CAD build for the part. Positions are in the model's coordinates, mm. A direction names the side the tool comes from. Coordinates: 2 decimals unless noted, no trailing zeros. Order: outer loops, then holes, each group sorted by start corner. A loop starts at its lowest first (then second) coordinate and runs counter-clockwise, first axis right, second up. Notation, with made-up numbers: M 51,7 L 109,7 A10 ccw 109,16 Z; hole C -27.75,4 d1. An arc over 180 degrees is marked long. One line per item, written item: value.
from build123d import *

# Parameters (mm, degrees)
BOSS_EXTRUDE1_DEPTH      = 90
CUT_EXTRUDE1_DEPTH       = 10
CHAMFER1_SIZE            = 1
CHAMFER1_EDGE_2_SIZE     = 1
CHAMFER1_EDGE_3_SIZE     = 1
CHAMFER1_EDGE_4_SIZE     = 1
CHAMFER1_EDGE_5_SIZE     = 1
CHAMFER1_EDGE_6_SIZE     = 1
BOSS_EXTRUDE2_DEPTH      = 2
BOSS_EXTRUDE2_DEPTH_BACK = 2
SKETCH2_R                = 1.75


with BuildPart() as part:
    # Sketch1 → Boss-Extrude1 (new body)
    with BuildSketch(Plane(origin=(0, 0, 0), x_dir=(0, 0, -1), z_dir=(1, 0, 0))):
        Polygon((3.464101615, -2), (3.464101615, 2), (0, 4), (-3.464101615, 2), (-3.464101615, -2), (0, -4), align=None)
    extrude(amount=BOSS_EXTRUDE1_DEPTH)

    # Sketch5 → Cut-Extrude1 (cut)
    with BuildSketch(Plane.ZY):
        with BuildLine():
            Line((1.404006351, -1.931810334), (2.375, -1.371206889))
            Line((2.375, -1.371206889), (2.375, -0.25))
            ThreePointArc((2.375, -0.25), (2.125, 0), (2.375, 0.25))
            Line((2.375, 0.25), (2.375, 1.371206889))
            Line((2.375, 1.371206889), (1.404006351, 1.931810334))
            ThreePointArc((1.404006351, 1.931810334), (1.0625, 1.840303983), (0.970993649, 2.181810334))
            Line((0.970993649, 2.181810334), (0, 2.742413779))
            Line((0, 2.742413779), (-0.970993649, 2.181810334))
            ThreePointArc((-0.970993649, 2.181810334), (-0.946018543, 2.121515095), (-0.9375, 2.056810334))
            ThreePointArc((-0.9375, 2.056810334), (-1.122795239, 1.815328877), (-1.404006351, 1.931810334))
            Line((-1.404006351, 1.931810334), (-2.375, 1.371206889))
            Line((-2.375, 1.371206889), (-2.375, 0.25))
            ThreePointArc((-2.375, 0.25), (-2.198223305, 0.176776695), (-2.125, 0))
            ThreePointArc((-2.125, 0), (-2.198223305, -0.176776695), (-2.375, -0.25))
            Line((-2.375, -0.25), (-2.375, -1.371206889))
            Line((-2.375, -1.371206889), (-1.404006351, -1.931810334))
            ThreePointArc((-1.404006351, -1.931810334), (-1.122795239, -1.815328877), (-0.9375, -2.056810334))
            ThreePointArc((-0.9375, -2.056810334), (-0.946018543, -2.121515095), (-0.970993649, -2.181810334))
            Line((-0.970993649, -2.181810334), (0, -2.742413779))
            Line((0, -2.742413779), (0.970993649, -2.181810334))
            ThreePointArc((0.970993649, -2.181810334), (1.0625, -1.840303983), (1.404006351, -1.931810334))
        make_face()
    extrude(amount=-CUT_EXTRUDE1_DEPTH, mode=Mode.SUBTRACT)

    # Chamfer1
    chamfer1_edges = [part.edges().sort_by_distance(p)[0] for p in [
        (45, -4, 0),
    ]]
    chamfer(chamfer1_edges, length=CHAMFER1_SIZE)

    # Chamfer1 edge 2
    chamfer1_edge_2_edges = [part.edges().sort_by_distance(p)[0] for p in [
        (45, -2, 3.464101615),
    ]]
    chamfer(chamfer1_edge_2_edges, length=CHAMFER1_EDGE_2_SIZE)

    # Chamfer1 edge 3
    chamfer1_edge_3_edges = [part.edges().sort_by_distance(p)[0] for p in [
        (45, 2, 3.464101615),
    ]]
    chamfer(chamfer1_edge_3_edges, length=CHAMFER1_EDGE_3_SIZE)

    # Chamfer1 edge 4
    chamfer1_edge_4_edges = [part.edges().sort_by_distance(p)[0] for p in [
        (45, 4, 0),
    ]]
    chamfer(chamfer1_edge_4_edges, length=CHAMFER1_EDGE_4_SIZE)

    # Chamfer1 edge 5
    chamfer1_edge_5_edges = [part.edges().sort_by_distance(p)[0] for p in [
        (45, 2, -3.464101615),
    ]]
    chamfer(chamfer1_edge_5_edges, length=CHAMFER1_EDGE_5_SIZE)

    # Chamfer1 edge 6
    chamfer1_edge_6_edges = [part.edges().sort_by_distance(p)[0] for p in [
        (45, -2, -3.464101615),
    ]]
    chamfer(chamfer1_edge_6_edges, length=CHAMFER1_EDGE_6_SIZE)

    # Sketch2 → Boss-Extrude2 (add, two sides: drawn at the far end of the back side and taken through both)
    with BuildSketch(Plane.XY.offset(-BOSS_EXTRUDE2_DEPTH_BACK)):
        with BuildLine():
            Line((90, 3.5), (97, 3.5))
            ThreePointArc((97, 3.5), (100.5, 0), (97, -3.5))
            Line((97, -3.5), (90, -3.5))
            Line((90, -3.5), (90, 3.5))
        make_face()
        with Locations((97, 0)):
            Circle(SKETCH2_R, mode=Mode.SUBTRACT)
    extrude(amount=BOSS_EXTRUDE2_DEPTH + BOSS_EXTRUDE2_DEPTH_BACK)


solid = part.part
Q1. Drill centre lines: line 1 along X through (y, z) = (-0.25, 0.5); line 2 along Y through (x, z) = (97, 1.1); line 3 along Z through (x, y) = (42, 2.25). Where is each one in solid material? Low to high.
Recorded:
line 1: x = 10 to 95.27, 98.73 to 100.49
line 2: y = -3.5 to -1.75, 1.75 to 3.5
line 3: z = -2.74 to 2.74
Q2. Slice it at A-A (x = 79). List the corners of the cut face in (y, z).
Recorded:
outline: M -3.5,-0.87 L -2.5,-2.6 L -1,-3.46 L 1,-3.46 L 2.5,-2.6 L 3.5,-0.87 L 3.5,0.87 L 2.5,2.6 L 1,3.46 L -1,3.46 L -2.5,2.6 L -3.5,0.87 Z
Q3. Slice it at B-B (x = 93.5). List the corners of the cut face in (y, z).
Recorded:
outline: M -3.5,-2 L 3.5,-2 L 3.5,2 L -3.5,2 Z
Q4. Mould opens along Y. For faces 6 (the face through (10, 0, 0)), 7 (the face through (44.37, 2.993, -1.744)), 8 (the face through (44.37, -2.993, 1.744)) say: released by +Y, released by -Y, zero draft, split by the parting line, or undercut.
Recorded:
face 6: undercut
face 7: released by +Y
face 8: released by -Y
Q5. Pin check, flat tips, straight feed: pin 1 Ø2.5 at (y, z) = (-1, 0) entering from -X; pin 2 Ø2 at (x, y) = (93, -0.5) entering from -Z; pin 3 Ø1.6 at (y, z) = (1.5, 3) entering from +X. Stop position of each tip, or through.
Recorded:
pin 1: stops at x = 10
pin 2: stops at z = -2
pin 3: stops at x = 90
Q6. Which spindle directions (+Z, -Z, +X, -X, +Y, -Y) get a long thin tool onto all of the face, cutting with end or side? Do faces 1 (the face through (44.37, 3.007, 1.72)), 2 (the face through (94, 0, -2)), 3 (the face through (94, 0, 2)), 4 (the face through (44.37, -3.007, -1.72)), 5 (the face through (44, 0, 3.464)). Say none if no direction does.
Recorded:
face 1: +Z, -X, +Y
face 2: -Z, +X, +Y, -Y
face 3: +Z, +X, +Y, -Y
face 4: -Z, -X, -Y
face 5: +Z, +X, -X, +Y, -Y
